from build123d import *

# Parameters (mm, degrees)
SKIZZE1_W                       = 90
SKIZZE1_H                       = 65
AUFSATZ_LINEAR_AUSTRAGEN1_DEPTH = 3
SKIZZE2_W                       = 20
SKIZZE2_H                       = 15
SCHNITT_LINEAR_AUSTRAGEN1_DEPTH = 1
SKIZZE3_R                       = 2.5
AUFSATZ_LINEAR_AUSTRAGEN2_DEPTH = 4
SKIZZE4_R                       = 1.364499713
SCHNITT_LINEAR_AUSTRAGEN2_DEPTH = 56.948637159
VERRUNDUNG1_R                   = 3
SKIZZE5_R                       = 2.25
SCHNITT_LINEAR_AUSTRAGEN3_DEPTH = 56.65294242
F_LLMUSTER1_OUTLINE_R           = 2.25
F_LLMUSTER1_DEPTH               = 3


# Read off the part's stored shape, not the designer's step: Füllmuster1
with BuildPart() as part:
    # Skizze1 → Aufsatz-Linear austragen1 (new body)
    with BuildSketch(Plane(origin=(0, 0, 0), x_dir=(1, 0, 0), z_dir=(0, 1, 0))):
        Rectangle(SKIZZE1_W, SKIZZE1_H)
    extrude(amount=AUFSATZ_LINEAR_AUSTRAGEN1_DEPTH)

    # Skizze2 → Schnitt-Linear austragen1 (cut)
    with BuildSketch(Plane(origin=(0, 3, 0), x_dir=(1, 0, 0), z_dir=(0, 1, 0))):
        with Locations((-35, 0)):
            Rectangle(SKIZZE2_W, SKIZZE2_H)
    extrude(amount=-SCHNITT_LINEAR_AUSTRAGEN1_DEPTH, mode=Mode.SUBTRACT)

    # Skizze3 → Aufsatz-Linear austragen2 (add)
    with BuildSketch(Plane(origin=(0, 3, 0), x_dir=(1, 0, 0), z_dir=(0, 1, 0))):
        with Locations(Location((-39, 24.5, 0), (0, 0, 270))):
            Circle(SKIZZE3_R)
        with Locations(Location((19.085512482, 24.5, 0), (0, 0, 270))):
            Circle(SKIZZE3_R)
        with Locations(Location((19.085512482, -24.5, 0), (0, 0, 270))):
            Circle(SKIZZE3_R)
        with Locations(Location((-39, -24.5, 0), (0, 0, 270))):
            Circle(SKIZZE3_R)
    extrude(amount=AUFSATZ_LINEAR_AUSTRAGEN2_DEPTH)

    # Skizze4 → Schnitt-Linear austragen2 (cut, through all)
    with BuildSketch(Plane(origin=(0, 7, 0), x_dir=(1, 0, 0), z_dir=(0, 1, 0))):
        with Locations(Location((19.085512482, 24.5, 0), (0, 0, 270))):
            Circle(SKIZZE4_R)
        with Locations(Location((-39, 24.5, 0), (0, 0, 270))):
            Circle(SKIZZE4_R)
        with Locations(Location((-39, -24.5, 0), (0, 0, 270))):
            Circle(SKIZZE4_R)
        with Locations(Location((19.085512482, -24.5, 0), (0, 0, 270))):
            Circle(SKIZZE4_R)
    extrude(amount=-SCHNITT_LINEAR_AUSTRAGEN2_DEPTH, mode=Mode.SUBTRACT)

    # Verrundung1
    verrundung1_edges = [part.edges().sort_by_distance(p)[0] for p in [
        (-45, 1.5, 32.5),
        (-45, 1.5, -32.5),
        (45, 1.5, -32.5),
        (45, 1.5, 32.5),
    ]]
    fillet(verrundung1_edges, radius=VERRUNDUNG1_R)

    # Skizze5 → Schnitt-Linear austragen3 (cut, through all)
    with BuildSketch(Plane(origin=(0, 3, 0), x_dir=(1, 0, 0), z_dir=(0, 1, 0))):
        with Locations(Location((-32, 28.5, 0), (0, 0, 270))):
            Circle(SKIZZE5_R)
    extrude(amount=-SCHNITT_LINEAR_AUSTRAGEN3_DEPTH, mode=Mode.SUBTRACT)

    # Füllmuster1 outline → Füllmuster1 (cut)
    with BuildSketch(Plane(origin=(0, 0, 0), x_dir=(1, 0, 0), z_dir=(0, 1, 0))):
        with Locations((40, 28.5)):
            Circle(F_LLMUSTER1_OUTLINE_R)
        with Locations((-32, -19.5)):
            Circle(F_LLMUSTER1_OUTLINE_R)
        with Locations((-40, 12.5)):
            Circle(F_LLMUSTER1_OUTLINE_R)
        with Locations((-40, -11.5)):
            Circle(F_LLMUSTER1_OUTLINE_R)
        with Locations((16, 4.5)):
            Circle(F_LLMUSTER1_OUTLINE_R)
        with Locations((16, -3.5)):
            Circle(F_LLMUSTER1_OUTLINE_R)
        with Locations((16, -11.5)):
            Circle(F_LLMUSTER1_OUTLINE_R)
        with Locations((8, 28.5)):
            Circle(F_LLMUSTER1_OUTLINE_R)
        with Locations((24, 4.5)):
            Circle(F_LLMUSTER1_OUTLINE_R)
        with Locations((24, -3.5)):
            Circle(F_LLMUSTER1_OUTLINE_R)
        with Locations((24, -11.5)):
            Circle(F_LLMUSTER1_OUTLINE_R)
        with Locations((16, 12.5)):
            Circle(F_LLMUSTER1_OUTLINE_R)
        with Locations((8, -11.5)):
            Circle(F_LLMUSTER1_OUTLINE_R)
        with Locations((8, -19.5)):
            Circle(F_LLMUSTER1_OUTLINE_R)
        with Locations((8, -27.5)):
            Circle(F_LLMUSTER1_OUTLINE_R)
        with Locations((0, 28.5)):
            Circle(F_LLMUSTER1_OUTLINE_R)
        with Locations((8, -3.5)):
            Circle(F_LLMUSTER1_OUTLINE_R)
        with Locations((8, 4.5)):
            Circle(F_LLMUSTER1_OUTLINE_R)
        with Locations((8, 12.5)):
            Circle(F_LLMUSTER1_OUTLINE_R)
        with Locations((8, 20.5)):
            Circle(F_LLMUSTER1_OUTLINE_R)
        with Locations((40, -11.5)):
            Circle(F_LLMUSTER1_OUTLINE_R)
        with Locations((40, -19.5)):
            Circle(F_LLMUSTER1_OUTLINE_R)
        with Locations((40, -27.5)):
            Circle(F_LLMUSTER1_OUTLINE_R)
        with Locations((32, 28.5)):
            Circle(F_LLMUSTER1_OUTLINE_R)
        with Locations((40, -3.5)):
            Circle(F_LLMUSTER1_OUTLINE_R)
        with Locations((40, 4.5)):
            Circle(F_LLMUSTER1_OUTLINE_R)
        with Locations((40, 12.5)):
            Circle(F_LLMUSTER1_OUTLINE_R)
        with Locations((40, 20.5)):
            Circle(F_LLMUSTER1_OUTLINE_R)
        with Locations((32, -11.5)):
            Circle(F_LLMUSTER1_OUTLINE_R)
        with Locations((32, -19.5)):
            Circle(F_LLMUSTER1_OUTLINE_R)
        with Locations((32, -27.5)):
            Circle(F_LLMUSTER1_OUTLINE_R)
        with Locations((24, 12.5)):
            Circle(F_LLMUSTER1_OUTLINE_R)
        with Locations((32, -3.5)):
            Circle(F_LLMUSTER1_OUTLINE_R)
        with Locations((32, 4.5)):
            Circle(F_LLMUSTER1_OUTLINE_R)
        with Locations((32, 12.5)):
            Circle(F_LLMUSTER1_OUTLINE_R)
        with Locations((32, 20.5)):
            Circle(F_LLMUSTER1_OUTLINE_R)
        with Locations((-16, -11.5)):
            Circle(F_LLMUSTER1_OUTLINE_R)
        with Locations((-16, -19.5)):
            Circle(F_LLMUSTER1_OUTLINE_R)
        with Locations((-16, -27.5)):
            Circle(F_LLMUSTER1_OUTLINE_R)
        with Locations((-24, 28.5)):
            Circle(F_LLMUSTER1_OUTLINE_R)
        with Locations((-16, -3.5)):
            Circle(F_LLMUSTER1_OUTLINE_R)
        with Locations((-16, 4.5)):
            Circle(F_LLMUSTER1_OUTLINE_R)
        with Locations((-16, 12.5)):
            Circle(F_LLMUSTER1_OUTLINE_R)
        with Locations((-16, 20.5)):
            Circle(F_LLMUSTER1_OUTLINE_R)
        with Locations((-24, -27.5)):
            Circle(F_LLMUSTER1_OUTLINE_R)
        with Locations((-32, 20.5)):
            Circle(F_LLMUSTER1_OUTLINE_R)
        with Locations((-32, 12.5)):
            Circle(F_LLMUSTER1_OUTLINE_R)
        with Locations((-32, -11.5)):
            Circle(F_LLMUSTER1_OUTLINE_R)
        with Locations((-24, -19.5)):
            Circle(F_LLMUSTER1_OUTLINE_R)
        with Locations((-24, -11.5)):
            Circle(F_LLMUSTER1_OUTLINE_R)
        with Locations((-24, 12.5)):
            Circle(F_LLMUSTER1_OUTLINE_R)
        with Locations((-24, 20.5)):
            Circle(F_LLMUSTER1_OUTLINE_R)
        with Locations((0, -11.5)):
            Circle(F_LLMUSTER1_OUTLINE_R)
        with Locations((0, -19.5)):
            Circle(F_LLMUSTER1_OUTLINE_R)
        with Locations((0, -27.5)):
            Circle(F_LLMUSTER1_OUTLINE_R)
        with Locations((-8, 28.5)):
            Circle(F_LLMUSTER1_OUTLINE_R)
        with Locations((0, -3.5)):
            Circle(F_LLMUSTER1_OUTLINE_R)
        with Locations((0, 4.5)):
            Circle(F_LLMUSTER1_OUTLINE_R)
        with Locations((0, 12.5)):
            Circle(F_LLMUSTER1_OUTLINE_R)
        with Locations((0, 20.5)):
            Circle(F_LLMUSTER1_OUTLINE_R)
        with Locations((-8, -11.5)):
            Circle(F_LLMUSTER1_OUTLINE_R)
        with Locations((-8, -19.5)):
            Circle(F_LLMUSTER1_OUTLINE_R)
        with Locations((-8, -27.5)):
            Circle(F_LLMUSTER1_OUTLINE_R)
        with Locations((-16, 28.5)):
            Circle(F_LLMUSTER1_OUTLINE_R)
        with Locations((-8, -3.5)):
            Circle(F_LLMUSTER1_OUTLINE_R)
        with Locations((-8, 4.5)):
            Circle(F_LLMUSTER1_OUTLINE_R)
        with Locations((-8, 12.5)):
            Circle(F_LLMUSTER1_OUTLINE_R)
        with Locations((-8, 20.5)):
            Circle(F_LLMUSTER1_OUTLINE_R)
    extrude(amount=F_LLMUSTER1_DEPTH, mode=Mode.SUBTRACT)


solid = part.part
Model file for the job. Use its own axes, mm. A direction names the side the tool comes from. Give positions to 0.01 mm unless a question says otherwise; leave off trailing zeros. Write each loop counter-clockwise with the first axis right and the second up, starting at its lowest first coordinate (ties: lowest second). Pieces come first, ordered by that corner, then holes. Notation, with made-up numbers: (12.5, -31) -> (57.5, -31) arc R14 cw to (57.5, -5) -> close; hole circle Ø5 at (-13.5, 35.25). An arc over 180 degrees is marked (long way). Write item = value, one per line.
(1) Mould opens along Z. For faces 1 (the face through (44.1, 1.52, -31.64)), 2 (the face through (-0.29, 1.48, -14.73)), 3 (the face through (-45, 1, 0)) say: released by +Z, released by -Z, zero draft, split by the parting line, or undercut.
Determined:
face_1 = released by -Z
face_2 = undercut
face_3 = zero draft
(2) Slice it at C-C, the plane z = -12.5. Give the number of separate pieces and of enclosed holes in the cut face, then the cut area to 4 significant figures.
Determined:
separate_pieces = 12
enclosed_holes = 0
area = 121.5 mm2
(3) Slice it at A-A, the plane z = -24.5. Give the cut face in (x, y), then the cut area to 3 significant figures.
Determined:
outline = (-45, 0) -> (-40.36, 0) -> (-40.36, 7) -> (-41.5, 7) -> (-41.5, 3) -> (-45, 3) -> close; (-37.64, 0) -> (17.72, 0) -> (17.72, 7) -> (16.59, 7) -> (16.59, 3) -> (-36.5, 3) -> (-36.5, 7) -> (-37.64, 7) -> close; (20.45, 0) -> (45, 0) -> (45, 3) -> (21.59, 3) -> (21.59, 7) -> (20.45, 7) -> close
area = 272 mm2
(4) Probe line 1 along Z through (x, y) = (16, 1.9); line 2 along X through (y, z) = (4.5, -23.5); line 3 along Z through (x, y) = (25.5, 1.5). List the from-to ranges inside material, lowest first.
Determined:
line_1 = -32.5 to -14.75, -10.25 to -6.75, -2.25 to 1.25, 5.75 to 9.25, 13.75 to 32.5
line_2 = -41.29 to -39.93, -38.07 to -36.71, 16.79 to 18.16, 20.01 to 21.38
line_3 = -32.5 to -14.18, -10.82 to -6.18, -2.82 to 1.82, 5.18 to 9.82, 13.18 to 32.5
(5) Tool access for faces 4 (the face through (-41.66, 1.48, 9.98)), 5 (the face through (17.56, 4.97, -26.48)): list every direction of +Z, -Z, +X, -X, +Y, -Y with a clear straight run to the whole face (end or side of a thin tool).
Determined:
face_4 = +Y, -Y
face_5 = +Y
(6) Flat gauge pins, fed straight in: P1, Ø5, axis at x = 40, z = 3.5, coming from the +Y side; P2, Ø2.5, axis at x = 32, z = 3.5, coming from the +Y side; P3, Ø4, axis at y = 6, z = -25, coming from the -X side. Where does each tip first touch, or does it go through?
Determined:
P1 = 3
P2 = through
P3 = -41.5
(7) Slice it at B-B, the plane x = -19.5. Give the cut face in (y, z), then the cut area to 3 significant figures.
Determined:
outline = (0, -32.5) -> (3, -32.5) -> (3, 32.5) -> (0, 32.5) -> close
area = 195 mm2
